Autodesk Inventor part; units mm, degrees
ref_plane "YZ Plane" through (0, 0, 0) normal (1, 0, 0) x (0, 1, 0)
ref_plane "XZ Plane" through (0, 0, 0) normal (0, 1, 0) x (-1, 0, 0)
ref_plane "XY Plane" through (0, 0, 0) normal (0, 0, 1) x (1, 0, 0)
sketch "Sketch1" plane through (0, 0, 0) normal (0, 0, 1) x (1, 0, 0)
  line L0 (-34.9037, 22.6593) -> (3.0963, 22.6593)
  line L1 (3.0963, 22.6593) -> (3.0963, -37.3407)
  line L2 (3.0963, -37.3407) -> (-34.9037, -37.3407)
  line L3 (-34.9037, -37.3407) -> (-34.9037, 22.6593)
  point P0 (0, 0)
  dimension "d0" = 38
  dimension "d1" = 60
extrude "Extrusion1" add sketch "Sketch1" along normal blind 5
sketch "Sketch2" plane through (0, 0, 5) normal (0, 0, 1) x (1, 0, 0)
  line L0 (3.0963, -37.3407) -> (3.0963, 22.6593)
  line L1 (3.0963, 22.6593) -> (-34.9037, 22.6593)
  line L2 (-34.9037, -37.3407) -> (3.0963, -37.3407)
  point P0 (0, 0)
  point P1 (-31.9037, 17.6593)
  point P2 (-1.9037, 17.6593)
  point P3 (-31.9037, -32.3407)
  point P4 (-1.9037, -32.3407)
  dimension "d4" = 30
  dimension "d5" = 30
  dimension "d6" = 5
  dimension "d7" = 5
  dimension "d8" = 5
  dimension "d9" = 5
  dimension "d10" = 5
  dimension "d11" = 5
hole "Hole1" at (-31.9037, 17.6593, 5) at (-1.9037, 17.6593, 5) at (-31.9037, -32.3407, 5) at (-1.9037, -32.3407, 5) direction (0, 0, -1) diameter 2 depth 10 tip angle 118
sketch "Sketch3" plane through (0, 0, 5) normal (0, 0, 1) x (1, 0, 0)
  line L0 (-28.9037, 20.6593) -> (-5.9037, 20.6593)
  line L1 (-5.9037, 20.6593) -> (-5.9037, -35.3407)
  line L2 (-5.9037, -35.3407) -> (-28.9037, -35.3407)
  line L3 (-28.9037, -35.3407) -> (-28.9037, 20.6593)
  line L4 (-32.9037, 12.6593) -> (-0.795, 12.6593)
  line L5 (-0.795, 12.6593) -> (-0.795, -27.3407)
  line L6 (-0.795, -27.3407) -> (-32.9037, -27.3407)
  line L7 (-32.9037, -27.3407) -> (-32.9037, 12.6593)
  line L8 (-34.9037, 22.6593) -> (-34.9037, -37.3407)
  line L9 (3.0963, -37.3407) -> (3.0963, 22.6593)
  line L10 (3.0963, 22.6593) -> (-34.9037, 22.6593)
  line L11 (-34.9037, -37.3407) -> (3.0963, -37.3407)
  point P0 (0, 0)
  point P1 (-28.9037, 12.6593)
  point P2 (-28.9037, -27.3407)
  point P3 (-5.9037, -27.3407)
  point P4 (-5.9037, 12.6593)
  dimension "d19" = 2
  dimension "d20" = 3.8913
  dimension "d21" = 2
  dimension "d22" = 2
  dimension "d23" = 6
  dimension "d24" = 9
  dimension "d25" = 10
  dimension "d26" = 10
extrude "Extrusion2" cut sketch "Sketch3" against normal blind 5 contours L0 L1 L4 L3 | L4 L1 L6 L3 | L3 L6 L7 L4 | L4 L5 L6 L1 | L6 L1 L2 L3
sketch "Sketch4" plane through (3.0963, -37.3407, 0) normal (1, 0, 0) x (0, 0, -1)
  line L0 (-5, 50) -> (-3, 50)
  line L1 (-3, 50) -> (-3, 38)
  line L2 (-3, 38) -> (-5, 38)
  line L3 (-5, 38) -> (-5, 50)
  line L4 (-5, 60) -> (-5, 0)
  line L5 (-5, 10) -> (-3, 10)
  line L6 (-3, 10) -> (-3, 22)
  line L7 (-3, 22) -> (-5, 22)
  line L8 (-5, 22) -> (-5, 10)
  line L9 (-5, 10) -> (0, 10)
  line L10 (-5, 50) -> (0, 50)
  point P0 (0, 37.3407)
  dimension "d29" = 12
  dimension "d30" = 12
  dimension "d31" = 0
  dimension "d32" = 2
extrude "Extrusion3" cut sketch "Sketch4" against normal blind 5
fillet "Fillet1" radius 5 2 edges at (3.0963, 22.6593, 2.5) (3.0963, -37.3407, 2.5)
sketch "Sketch5" plane through (0, 0, 0) normal (0, 0, -1) x (-1, 0, 0)
  line L0 (5.9037, 20.6593) -> (28.9037, 20.6593)
  line L1 (13.9037, 20.6593) -> (11.9037, 20.6593)
  line L2 (11.9037, 20.6593) -> (11.9037, -35.3407)
  line L3 (11.9037, -35.3407) -> (13.9037, -35.3407)
  line L4 (13.9037, -35.3407) -> (13.9037, 20.6593)
  line L5 (-3.0963, -32.3407) -> (-3.0963, 17.6593)
  line L6 (28.9037, -35.3407) -> (5.9037, -35.3407)
  point P0 (0, 0)
  dimension "d36" = 15
  dimension "d37" = 2
extrude "Extrusion4" add sketch "Sketch5" against normal blind 3
fillet "Fillet2" radius 5 4 edges at (-28.9037, 12.6593, 2.5) (-28.9037, -27.3407, 2.5) (-5.9037, -27.3407, 2.5) (-5.9037, 12.6593, 2.5)
fillet "Fillet3" radius 2 4 edges at (-13.9037, 20.6593, 1.5) (-11.9037, 20.6593, 1.5) (-11.9037, -35.3407, 1.5) (-13.9037, -35.3407, 1.5)
properties part number "atx-adapter_cable-press"
Design review of the part built by this model. Coordinates are the model's own, in mm. A direction names the side the tool comes from. Round coordinates to 2 decimals unless told otherwise and drop trailing zeros. Write each loop counter-clockwise with the first axis right and the second up, starting at its lowest first coordinate (ties: lowest second). Pieces come first, ordered by that corner, then holes. Notation, with made-up numbers: (-10, -6.5) - (20, -6.5) arc R31 ccw to (20, 21.5) - close; hole circle Ø6 at (33.25, 12.25). An arc over 180 degrees is marked (long way). Return JSON: item names as keys, results as strings. Group by question number.
Item 1: We need section A-A on x = -7. Write out the cut boundary in (y, z).
Item 2: Insertion check: P1, Ø2, axis at x = 1.5, z = 3, coming from the -Y side (3 decimals); P2, Ø2.5, axis at y = 19.5, z = 1.5, coming from the +X side; P3, Ø1.9, axis at x = 1.5, y = -20.5, coming from the +Z side. Each pin has a flat end and moves straight along its axis. Give the tip position at first contact, or say it passes through.
Item 3: The part is to be moulded in two halves that separate along X. For faces 4 (the face through (-34, -7, 5)), 5 (the face through (3.096, -7, 2)), 6 (the face through (-13.904, -8, 1)), say which applies: pulls with the +X half, pulls with the -X half, needs draft (parallel to the pull), parting line crosses it, or undercut.
Item 4: For probe 1 along X at (y, z) = (-27, 1.95) (3 decimals); probe 2 along X at (y, z) = (-8, 4.2) (3 decimals); probe 3 along Y at (x, z) = (-21, 3.7), list the stretches that pass through material, from the lowest coordinate up. Write a range as [from, to].
Item 5: Machinability: for faces 1 (the face through (-13, -7, 3)), 2 (the face through (-30.06, 14.36, 2.54)), 3 (the face through (1, 7, 3)), which of the approach directions +Z, -Z, +X, -X, +Y, -Y give a long, thin tool a straight path to every point of the face, cutting with its end or side? Answer none if there is none.
Item 6: We need section B-B on y = -14. Write out the cut boundary in (x, z) (3 decimals).
Item 7: We need section C-C on z = 4.1. Write out the cut boundary in (x, y) (3 decimals), and give its area (3 significant figures).
Item 8: We need section D-D on x = -13. Write out the cut boundary in (y, z).
Model answer:
{
 "1": {"outline": "(-37.34, 0) - (-35.34, 0) - (-35.34, 5) - (-37.34, 5) - close; (20.66, 0) - (22.66, 0) - (22.66, 5) - (20.66, 5) - close"},
 "2": {"P1": "stops at y = -36.725", "P2": "stops at x = 3.06", "P3": "stops at z = 3"},
 "3": {"face 4": "needs draft", "face 5": "pulls with the +X half", "face 6": "undercut"},
 "4": {"probe 1": "x = [-34.904, -32.904], [-13.904, -11.904], [-0.795, 3.096]", "probe 2": "x = [-34.904, -32.904], [-0.795, 3.096]", "probe 3": "y = [-37.34, -35.34], [20.66, 22.66]"},
 "5": {"face 1": "+Z", "face 2": "+Z, -Z", "face 3": "+Z, +X"},
 "6": {"outline": "(-34.904, 0) - (-32.904, 0) - (-32.904, 5) - (-34.904, 5) - close; (-13.904, 0) - (-11.904, 0) - (-11.904, 3) - (-13.904, 3) - close; (-0.795, 0) - (3.096, 0) - (3.096, 5) - (-0.795, 5) - close"},
 "7": {"outline": "(-34.904, -37.341) - (-1.904, -37.341) arc R5 ccw to (3.096, -32.341) - (3.096, -27.341) - (-0.904, -27.341) arc R5 ccw to (-5.904, -32.341) - (-5.904, -35.341) - (-28.904, -35.341) - (-28.904, -32.24) arc R5 ccw to (-32.904, -27.341) - (-32.904, 12.659) arc R5 ccw to (-28.904, 17.558) - (-28.904, 20.659) - (-5.904, 20.659) - (-5.904, 17.659) arc R5 ccw to (-0.904, 12.659) - (3.096, 12.659) - (3.096, 17.659) arc R5 ccw to (-1.904, 22.659) - (-34.904, 22.659) - close; (-0.795, -15.341) - (3.096, -15.341) - (3.096, 0.659) - (-0.795, 0.659) - close; hole circle Ø2 at (-31.904, -32.341); hole circle Ø2 at (-31.904, 17.659); hole circle Ø2 at (-1.904, -32.341); hole circle Ø2 at (-1.904, 17.659)", "area": "490 mm²"},
 "8": {"outline": "(-37.34, 0) - (22.66, 0) - (22.66, 5) - (20.66, 5) - (20.66, 3) - (-35.34, 3) - (-35.34, 5) - (-37.34, 5) - close"}
}
